from build123d import *

# Parameters (mm, degrees)
IZIM1_R            = 30.75
TABAN_FLAN_1_DEPTH = 40


# Sheet-metal steps are written as plain solids
with BuildPart() as part:
    # Çizim1 → Taban-Flanş1 (new body)
    with BuildSketch(Plane.XY):
        with BuildLine():
            Line((-1.643398768, 91.658785331), (231.87468677, 210.823863864))
            ThreePointArc((231.87468677, 210.823863864), (256.473387586, 210.2990154), (279.460662471, 201.526516265))
            ThreePointArc((279.460662471, 201.526516265), (342.491227066, 147.22978074), (379.677674371, 72.810994814))
            ThreePointArc((379.677674371, 72.810994814), (375.525370831, 20.220941214), (339.489037745, -18.306166907))
            ThreePointArc((339.489037745, -18.306166907), (330.00144074, -17.604735784), (321.25415431, -13.864216747))
            ThreePointArc((321.25415431, -13.864216747), (316.568149269, -9.137053114), (315.500028304, -2.567134022))
            Line((315.500028304, -2.567134022), (315.804951466, 0.498028518))
            ThreePointArc((315.804951466, 0.498028518), (275.813280207, 66.354649224), (208.223919967, 29.366723581))
            ThreePointArc((208.223919967, 29.366723581), (204.280862876, 21.941440766), (199.589645635, 14.964693321))
            ThreePointArc((199.589645635, 14.964693321), (189.567794587, 8.489124316), (177.959719616, 5.728130318))
            ThreePointArc((177.959719616, 5.728130318), (170.039190968, 4.902214912), (162.171757217, 3.669171324))
            Line((162.171757217, 3.669171324), (63.894243865, -16.687773846))
            ThreePointArc((63.894243865, -16.687773846), (52.087429233, -18.756679073), (40.128679606, -19.57493818))
            ThreePointArc((40.128679606, -19.57493818), (-13.999894405, 23.558211566), (-1.643398768, 91.658785331))
        make_face()
        with Locations((47.296813478, 47.891327559)):
            Circle(IZIM1_R, mode=Mode.SUBTRACT)
        with Locations((220.432800905, 137.607155914)):
            Circle(IZIM1_R, mode=Mode.SUBTRACT)
    extrude(amount=-TABAN_FLAN_1_DEPTH)


solid = part.part
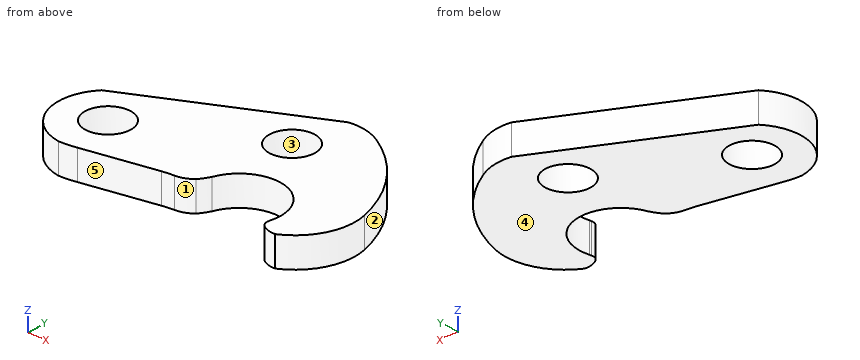
Part model, mm, in its own coordinate system. Face numbers are marked on the shaded views. A direction names the side the tool comes from. Round coordinates to 2 decimals unless told otherwise and drop trailing zeros. Write each loop counter-clockwise with the first axis right and the second up, starting at its lowest first coordinate (ties: lowest second). Pieces come first, ordered by that corner, then holes. Notation, with made-up numbers: (42.25, 5) - (99.25, 5) arc R28 ccw to (99.25, 27) - close; hole circle Ø4 at (-5, -37). An arc over 180 degrees is marked (long way). Use CSV: the item, a comma, the result in double quotes.
Item 1: Pull direction Y, two halves, no side cores. Call the marked faces 1, 2 and 3: pulls with the +Y half, pulls with the -Y half, needs draft (parallel to the pull), parting line crosses it, or undercut.
Results list:
face 1,"pulls with the -Y half"
face 2,"pulls with the +Y half"
face 3,"undercut"
Item 2: Wall check: L1, parallel to X at y = 74.5, z = -4.5; L2, parallel to X at y = 62.5, z = -6; L3, parallel to Y at x = 30.5, z = -31.5. Give the ranges that are in metal, low to high.
Results list:
L1,"x = -12.57 to 31.88, 62.71 to 379.21"
L2,"x = -16.56 to 20.24, 74.36 to 236.69, 286.04 to 381.68"
L3,"y = -17.55 to 22.13, 73.65 to 108.06"
Item 3: Slice it at B-B, the plane x = 212. Write the cut outline in (y, z).
Results list:
outline,"(38.42, -40) - (108.04, -40) - (108.04, 0) - (38.42, 0) - close; (167.18, -40) - (200.68, -40) - (200.68, 0) - (167.18, 0) - close"
Item 4: Slice it at D-D, the plane y = 143. Write the cut outline in (x, z).
Results list:
outline,"(98.97, -40) - (190.16, -40) - (190.16, 0) - (98.97, 0) - close; (250.71, -40) - (345.7, -40) - (345.7, 0) - (250.71, 0) - close"
Item 5: Tool access for the marked faces 4 and 5: list every direction of +Z, -Z, +X, -X, +Y, -Y with a clear straight run to the whole face (end or side of a thin tool).
Results list:
face 4,"-Z, +X, -X, +Y, -Y"
face 5,"+Z, -Z, -Y"
Item 6: Slice it at C-C, the plane z = -16.5. Write the cut outline in (x, y), then the cut area to 3 significant figures.
Results list:
outline,"(-1.64, 91.66) arc R67.45 ccw to (40.13, -19.57) arc R114.05 ccw to (63.89, -16.69) - (162.17, 3.67) arc R154.46 cw to (177.96, 5.73) arc R35.25 ccw to (199.59, 14.96) arc R81.03 ccw to (208.22, 29.37) arc R55.75 cw to (315.8, 0.5) - (315.5, -2.57) arc R10.91 ccw to (321.25, -13.86) arc R28.93 ccw to (339.49, -18.31) arc R79.86 ccw to (379.68, 72.81) arc R211.3 ccw to (279.46, 201.53) arc R72.04 ccw to (231.87, 210.82) - close; hole circle Ø61.5 at (47.3, 47.89); hole circle Ø61.5 at (220.43, 137.61)"
area,"51,200 mm²"
Item 7: Slice it at A-A, the plane y = 63. Write the cut outline in (x, z).
Results list:
outline,"(-16.45, -40) - (20.51, -40) - (20.51, 0) - (-16.45, 0) - close; (74.08, -40) - (237.73, -40) - (237.73, 0) - (74.08, 0) - close; (285, -40) - (381.62, -40) - (381.62, 0) - (285, 0) - close"
Item 8: Flat gauge pins, fed straight in: P1, Ø1, axis at y = 147.5, z = -35, coming from the +X side; P2, Ø1, axis at y = 115, z = -26, coming from the -X side; P3, Ø10, axis at x = 106, z = -28.5, coming from the -Y side. Where does each tip first touch, or does it go through?
Results list:
P1,"stops at x = 342.67"
P2,"stops at x = 43.12"
P3,"stops at y = -9"
